from build123d import *

# Parameters (mm, degrees)
EXTRUDE_2_DEPTH     = 68
SKETCH_2_W          = 5
SKETCH_2_H          = 58
EXTRUDE_3_DEPTH     = 20
CUT_EXTRUDE_1_DEPTH = 20
FILLET_1_R          = 4
SKETCH_4_W          = 68
SKETCH_4_H          = 3
EXTRUDE_4_DEPTH     = 8
CHAMFER_1_SIZE      = 2
CUT_EXTRUDE_3_DEPTH = 8
CUT_EXTRUDE_START   = -2.5
CUT_EXTRUDE_4_DEPTH = 2.5


with BuildPart() as part:
    # 草图1 → 凸台-拉伸2 (new body)
    with BuildSketch(Plane(origin=(0, 0, 0), x_dir=(0, 0, -1), z_dir=(1, 0, 0))):
        Polygon((0, 0), (-68, 0), (-68, 5), (-10, 5), (-10, 20), (0, 20), align=None)
    extrude(amount=EXTRUDE_2_DEPTH)

    # 草图2 → 凸台-拉伸3 (add)
    with BuildSketch(Plane(origin=(0, 5, 0), x_dir=(1, 0, 0), z_dir=(0, 1, 0))):
        with Locations((65.5, -39)):
            Rectangle(SKETCH_2_W, SKETCH_2_H)
        with Locations((2.5, -39)):
            Rectangle(SKETCH_2_W, SKETCH_2_H)
    extrude(amount=EXTRUDE_3_DEPTH)

    # 草图3 → 切除-拉伸1 (cut)
    with BuildSketch(Plane(origin=(0, 0, 0), x_dir=(-1, 0, 0), z_dir=(0, 0, -1))):
        with BuildLine():
            Line((-58, 14.75), (-43, 14.75))
            ThreePointArc((-43, 14.75), (-40.25, 12), (-43, 9.25))
            Line((-43, 9.25), (-58, 9.25))
            ThreePointArc((-58, 9.25), (-60.75, 12), (-58, 14.75))
        make_face()
        with BuildLine():
            Line((-25, 14.75), (-10, 14.75))
            ThreePointArc((-10, 14.75), (-7.25, 12), (-10, 9.25))
            Line((-10, 9.25), (-25, 9.25))
            ThreePointArc((-25, 9.25), (-27.75, 12), (-25, 14.75))
        make_face()
    extrude(amount=-CUT_EXTRUDE_1_DEPTH, mode=Mode.SUBTRACT)

    # 圆角1
    fillet_1_edges = [part.edges().sort_by_distance(p)[0] for p in [
        (34, 0, 0),
    ]]
    fillet(fillet_1_edges, radius=FILLET_1_R)

    # 草图4 → 凸台-拉伸4 (add)
    with BuildSketch(Plane(origin=(0, 25, 0), x_dir=(1, 0, 0), z_dir=(0, 1, 0))):
        with Locations((34, -69.5)):
            Rectangle(SKETCH_4_W, SKETCH_4_H)
    extrude(amount=-EXTRUDE_4_DEPTH)

    # 倒角1
    chamfer_1_edges = [part.edges().sort_by_distance(p)[0] for p in [
        (68, 21, 71),
        (0, 21, 71),
        (68, 22.5, 10),
        (63, 22.5, 10),
        (65.5, 25, 10),
        (5, 22.5, 10),
        (0, 22.5, 10),
        (2.5, 25, 10),
        (0, 8.5, 68),
        (68, 8.5, 68),
    ]]
    chamfer(chamfer_1_edges, length=CHAMFER_1_SIZE)

    # 草图5 → 切除-拉伸3 (cut)
    with BuildSketch(Plane.XZ):
        with BuildLine():
            Line((8, 17), (23, 17))
            ThreePointArc((23, 17), (25.5, 14.5), (23, 12))
            Line((23, 12), (8, 12))
            ThreePointArc((8, 12), (5.5, 14.5), (8, 17))
        make_face()
        with BuildLine():
            Line((45, 17), (60, 17))
            ThreePointArc((60, 17), (62.5, 14.5), (60, 12))
            Line((60, 12), (45, 12))
            ThreePointArc((45, 12), (42.5, 14.5), (45, 17))
        make_face()
    extrude(amount=-CUT_EXTRUDE_3_DEPTH, mode=Mode.SUBTRACT)

    # 草图7 → 切除-拉伸4 (cut)
    with BuildSketch(Plane(origin=(0, 5, 0), x_dir=(1, 0, 0), z_dir=(0, 1, 0)).offset(CUT_EXTRUDE_START)):
        with BuildLine():
            Line((23, -18.2), (8, -18.2))
            Line((8, -18.2), (8, -17))
            Line((8, -17), (23, -17))
            ThreePointArc((23, -17), (25.5, -14.5), (23, -12))
            Line((23, -12), (8, -12))
            Line((8, -12), (8, -10.8))
            Line((8, -10.8), (23, -10.8))
            ThreePointArc((23, -10.8), (26.7, -14.5), (23, -18.2))
        make_face()
        with BuildLine():
            Line((45, -10.8), (60, -10.8))
            Line((60, -10.8), (60, -12))
            Line((60, -12), (45, -12))
            ThreePointArc((45, -12), (42.5, -14.5), (45, -17))
            Line((45, -17), (60, -17))
            Line((60, -17), (60, -18.2))
            Line((60, -18.2), (45, -18.2))
            ThreePointArc((45, -18.2), (41.3, -14.5), (45, -10.8))
        make_face()
    extrude(amount=CUT_EXTRUDE_4_DEPTH, mode=Mode.SUBTRACT)


solid = part.part
Verification items for the finished model (mm, model axes). A direction names the side the tool comes from. Give positions to 0.01 mm unless a question says otherwise; leave off trailing zeros. Loops run counter-clockwise (first coordinate to the right, second up) from the corner with the lowest first, then second, coordinate; pieces in that order, holes last.
1) Sectioned sample at B-B, the plane x = 18.5. Enter the section's corners in (y, z), then the cut area to 3 significant figures.
2) Draft check along Z on faces 5 (the flat face through (53, 1, 12)), 6 (the cylindrical face through (60.75, 11.94, 4.93)), 7 (the flat face through (15, 1, 17)), 8 (the flat face through (1, 22, 11)). Enter one of: pulls with the +Z half, pulls with the -Z half, needs draft (parallel to the pull), parting line crosses it, or undercut.
3) Set-up check for faces 1 (the cylindrical face through (41.3, 3.7, 14.6)), 2 (the flat face through (34, 5, 39)), 3 (the cylindrical face through (40.25, 12.06, 4.93)), 4 (the flat face through (52, 1, 17)): record each of +Z, -Z, +X, -X, +Y, -Y from which the full face is reachable in a straight line by a thin tool's end or side.
4) Sectioned sample at C-C, the plane y = 12. Enter the section's corners in (x, z).
5) Sectioned sample at A-A, the plane z = 14.5. Enter the section's corners in (x, y), then the cut area to 3 significant figures.
6) Thickness scan on line 1 along X through (y, z) = (18.75, 63); line 2 along Z through (x, y) = (41, 19.75); line 3 along Y through (x, z) = (29, 53.5). Record the ranges inside material, lowest first.
7) Sectioned sample at D-D, the plane z = 65. Enter the section's corners in (x, y), then the cut area to 3 significant figures.
8) Depth check by flat-ended pin: pin 1 Ø3 at (x, z) = (41, 38) entering from +Y; pin 2 Ø2 at (x, y) = (54.5, 1.5) entering from +Z; pin 3 Ø8 at (x, z) = (17, 3) entering from +Y. Enter the tip coordinate at first touch or a pass-through.
Answers:
1. outline: (0, 4) arc R4 ccw to (4, 0) - (9.25, 0) - (9.25, 10) - (5, 10) - (5, 10.8) - (2.5, 10.8) - (2.5, 12) - (0, 12) - close; (0, 17) - (2.5, 17) - (2.5, 18.2) - (5, 18.2) - (5, 68) - (0, 68) - close; (14.75, 0) - (20, 0) - (20, 10) - (14.75, 10) - close; (17, 68) - (25, 68) - (25, 71) - (17, 71) - close
1. area: 425 mm2
2. face 5: undercut
2. face 6: needs draft
2. face 7: undercut
2. face 8: pulls with the -Z half
3. face 1: +Y
3. face 2: +Z, +Y
3. face 3: +Z, -Z
3. face 4: +Y, -Y
4. outline: (0, 0) - (7.25, 0) - (7.25, 10) - (5, 10) - (5, 68) - (2, 68) - (0, 66) - close; (27.75, 0) - (40.25, 0) - (40.25, 10) - (27.75, 10) - close; (60.75, 0) - (68, 0) - (68, 66) - (66, 68) - (63, 68) - (63, 10) - (60.75, 10) - close
5. outline: (0, 0) - (5.5, 0) - (5.5, 5) - (5, 5) - (5, 25) - (0, 25) - close; (25.5, 0) - (42.5, 0) - (42.5, 2.5) - (41.3, 2.5) - (41.3, 5) - (26.7, 5) - (26.7, 2.5) - (25.5, 2.5) - close; (62.5, 0) - (68, 0) - (68, 25) - (63, 25) - (63, 5) - (62.5, 5) - close
5. area: 334 mm2
6. line 1: x = 0 to 5, 63 to 68
6. line 2: z = 0 to 10, 68 to 71
6. line 3: y = 0 to 5
7. outline: (0, 0) - (68, 0) - (68, 25) - (63, 25) - (63, 5) - (5, 5) - (5, 25) - (0, 25) - close
7. area: 540 mm2
8. pin 1: stops at y = 5
8. pin 2: stops at z = 68
8. pin 3: stops at y = 20
